Part model, mm, in its own coordinate system. Face numbers are marked on the shaded views. A direction names the side the tool comes from. Coordinates: 2 decimals unless noted, no trailing zeros. Write each loop counter-clockwise with the first axis right and the second up, starting at its lowest first coordinate (ties: lowest second). Pieces come first, ordered by that corner, then holes. Notation, with made-up numbers: (68, 18) -> (104, 18) arc R17 ccw to (104, 48) -> close; hole circle Ø4 at (-9.5, -15). An arc over 180 degrees is marked (long way). Write item = value, one per line. Start each with the question number.
Q1. Band-saw the part on B-B, the plane z = -0.25. List the corners of the cut face in (x, y), plus the area to 3 significant figures.
Q2. Band-saw the part on D-D, the plane x = 5. List the corners of the cut face in (y, z).
Q3. Tool access for the marked faces 5 and 6: list every direction of +Z, -Z, +X, -X, +Y, -Y with a clear straight run to the whole face (end or side of a thin tool).
Q4. Band-saw the part on C-C, the plane y = -1.25. List the corners of the cut face in (x, z), plus the area to 3 significant figures.
Q5. Probe line 1 (Z direction, x = 22, y = 2.75); line 2 (X direction, y = -3.75, z = -5.25); line 3 (Y direction, x = 19, z = 4). List the from-to ranges inside material, lowest first.
Q6. Pull direction Z, two halves, no side cores. Call the marked faces 1, 2, 3 and 4: released by +Z, released by -Z, zero draft, split by the parting line, or undercut.
Q7. Band-saw the part on A-A, the plane y = 1.25. List the corners of the cut face in (x, z), plus the area to 3 significant figures.
Q8. Pin check, flat tips, straight feed: P1, Ø6, axis at x = 25, y = 4, coming from the -Z side; P2, Ø1.5, axis at x = 27.5, y = 0.5, coming from the +Z side; P3, Ø1.5, axis at x = 10, y = 6, coming from the -Z side. Stop position of each tip, or through.
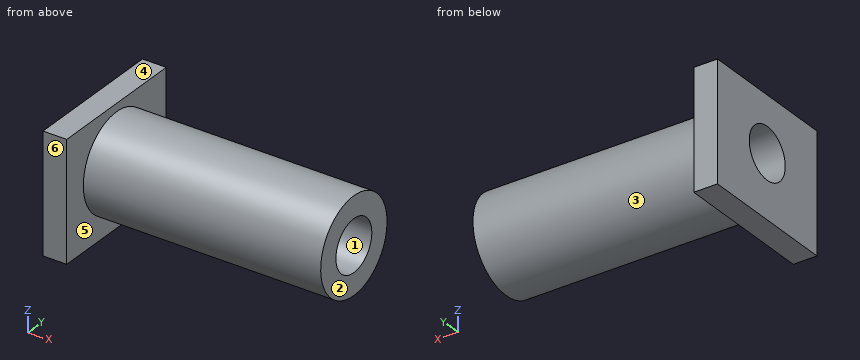
from build123d import *

# Parameters (mm, degrees)
SKETCH1_W           = 18
SKETCH1_H           = 15
SKETCH1_R           = 3.25
BOSS_EXTRUDE1_DEPTH = 3
SKETCH2_R           = 6
SKETCH2_R_2         = 3.25
BOSS_EXTRUDE2_DEPTH = 30


with BuildPart() as part:
    # Sketch1 → Boss-Extrude1 (new body)
    with BuildSketch(Plane.YZ):
        with Locations((2.662827036, 1.188789176)):
            Rectangle(SKETCH1_W, SKETCH1_H)
        with Locations(Location((2.662827036, 1.688789176, 0), (0, 0, 270))):
            Circle(SKETCH1_R, mode=Mode.SUBTRACT)
    extrude(amount=BOSS_EXTRUDE1_DEPTH)

    # Sketch2 → Boss-Extrude2 (add)
    with BuildSketch(Plane.YZ.offset(3)):
        with Locations(Location((2.662827036, 1.688789176, 0), (0, 0, 270))):
            Circle(SKETCH2_R)
        with Locations(Location((2.662827036, 1.688789176, 0), (0, 0, 270))):
            Circle(SKETCH2_R_2, mode=Mode.SUBTRACT)
    extrude(amount=BOSS_EXTRUDE2_DEPTH)


solid = part.part
Ans:
q1.outline = (0, -6.34) -> (3, -6.34) -> (3, -3.02) -> (33, -3.02) -> (33, 0.05) -> (0, 0.05) -> close; (0, 5.27) -> (33, 5.27) -> (33, 8.34) -> (3, 8.34) -> (3, 11.66) -> (0, 11.66) -> close
q1.area = 223 mm2
q2.outline = circle Ø12 at (2.66, 1.69); hole circle Ø6.5 at (2.66, 1.69)
q3.face_5 = +X
q3.face_6 = +Z, -Z, +X, -X, -Y
q4.outline = (0, -6.31) -> (3, -6.31) -> (3, -2.86) -> (33, -2.86) -> (33, 6.24) -> (3, 6.24) -> (3, 8.69) -> (0, 8.69) -> close
q4.area = 318 mm2
q5.line_1 = -4.31 to -1.56, 4.94 to 7.69
q5.line_2 = 0 to 3
q5.line_3 = -2.87 to 0.38, 4.95 to 8.2
q6.face_1 = undercut
q6.face_2 = zero draft
q6.face_3 = split by the parting line
q6.face_4 = released by +Z
q7.outline = (0, -6.31) -> (3, -6.31) -> (3, -4.14) -> (33, -4.14) -> (33, -1.24) -> (0, -1.24) -> close; (0, 4.62) -> (33, 4.62) -> (33, 7.52) -> (3, 7.52) -> (3, 8.69) -> (0, 8.69) -> close
q7.area = 202 mm2
q8.P1 = -4.31
q8.P2 = 7.52
q8.P3 = -3.72
